Source: CAD feature listing. Evaluate the final solid. Frame: model axes, mm. A direction names the side the tool comes from. Coordinates: 2 decimals unless noted, no trailing zeros. Loops run counter-clockwise (first coordinate to the right, second up) from the corner with the lowest first, then second, coordinate; pieces in that order, holes last. Notation, with made-up numbers: (64, 65.5) -> (83, 65.5) arc R25 ccw to (83, 79.5) -> close; hole circle Ø3 at (-13, -1.75). An arc over 180 degrees is marked (long way). Answer as CSV lines item,"result".
from build123d import *

# Parameters (mm, degrees)
F0_R     = 0.825
F0_R_2   = 7.825
F0_W     = 2.625
F0_H     = 2.7
F1_DEPTH = 1.6
F0_R_3   = 6.175
F2_DEPTH = 13.8
F3_DEPTH = 11.65
F4_DEPTH = 3.1
F5_W     = 0.8
F5_H     = 0.8
F6_DEPTH = 2.4
F8_DEPTH = 0.8
F9_DEPTH = 5
F10_R    = 0.3


with BuildPart() as f1:
    # F0 (on Top) → F1 (new body)
    with BuildSketch(Plane.XY):
        Polygon((22.85, -10.65), (22.85, 10.65), (5.25, 10.65), (5.25, 7.95), (2.625, 7.95), (0, 7.95), (-2.625, 7.95), (-5.25, 7.95), (-5.25, 10.65), (-22.85, 10.65), (-22.85, -10.65), align=None)
        with Locations((-21.125, -8.675)):
            Circle(F0_R, mode=Mode.SUBTRACT)
        with BuildLine():
            ThreePointArc((-4.1107536526, -10.25), (-6.4607536526, -7.9), (-4.1107536526, -5.55))
            Line((-4.1107536526, -5.55), (4.1107536526, -5.55))
            ThreePointArc((4.1107536526, -5.55), (6.4607536526, -7.9), (4.1107536526, -10.25))
            Line((4.1107536526, -10.25), (-4.1107536526, -10.25))
        make_face(mode=Mode.SUBTRACT)
        with Locations((21.125, -8.675)):
            Circle(F0_R, mode=Mode.SUBTRACT)
        with Locations((-13.025, 0)):
            Circle(F0_R_2, mode=Mode.SUBTRACT)
        with Locations((-21.125, 8.675)):
            Circle(F0_R, mode=Mode.SUBTRACT)
        with Locations((13.025, 0)):
            Circle(F0_R_2, mode=Mode.SUBTRACT)
        with Locations((21.125, 8.675)):
            Circle(F0_R, mode=Mode.SUBTRACT)
        with Locations((-3.9375, 9.3)):
            Rectangle(F0_W, F0_H)
        with Locations((-1.3125, 9.3)):
            Rectangle(F0_W, F0_H)
        with Locations((1.3125, 9.3)):
            Rectangle(F0_W, F0_H)
        with Locations((3.9375, 9.3)):
            Rectangle(F0_W, F0_H)
    extrude(amount=F1_DEPTH)

    # F0 (on Top) → F2 (join)
    with BuildSketch(Plane.XY):
        with Locations((13.025, 0)):
            Circle(F0_R_2)
        with Locations((13.025, 0)):
            Circle(F0_R_3, mode=Mode.SUBTRACT)
        with Locations((-13.025, 0)):
            Circle(F0_R_2)
        with Locations((-13.025, 0)):
            Circle(F0_R_3, mode=Mode.SUBTRACT)
    extrude(amount=F2_DEPTH)

    # F0 (on Top) → F3 (join)
    with BuildSketch(Plane.XY):
        with Locations((-13.025, 0)):
            Circle(F0_R_3)
        with Locations((13.025, 0)):
            Circle(F0_R_3)
    extrude(amount=F3_DEPTH)

    # F0 (on Top) → F4 (join)
    with BuildSketch(Plane.XY):
        with Locations((-3.9375, 9.3)):
            Rectangle(F0_W, F0_H)
        with Locations((-1.3125, 9.3)):
            Rectangle(F0_W, F0_H)
        with Locations((1.3125, 9.3)):
            Rectangle(F0_W, F0_H)
        with Locations((3.9375, 9.3)):
            Rectangle(F0_W, F0_H)
    extrude(amount=-F4_DEPTH)

    # F5 (on face) → F6 (join)
    with BuildSketch(Plane(origin=(0, 0, -3.1), x_dir=(1, 0, 0), z_dir=(0, 0, -1))):
        with Locations((-3.9375, -9.3)):
            Rectangle(F5_W, F5_H)
        with Locations((-1.3125100119, -9.3)):
            Rectangle(F5_W, F5_H)
        with Locations((1.3124799761, -9.3)):
            Rectangle(F5_W, F5_H)
        with Locations((3.9374699642, -9.3)):
            Rectangle(F5_W, F5_H)
    extrude(amount=F6_DEPTH)

    # F7 (on face) → F8 (join)
    with BuildSketch(Plane(origin=(0, 0, -5.5), x_dir=(1, 0, 0), z_dir=(0, 0, -1))):
        Polygon((-4.3375, -8.9), (-4.3375, -9.7), (-4.3375, -16.8), (-3.5375, -16.8), (-3.5375, -9.7), (-3.5375, -8.9), align=None)
        Polygon((-1.7125100119, -8.9), (-1.7125100119, -9.7), (-1.7125100119, -16.8), (-0.9125100119, -16.8), (-0.9125100119, -9.7), (-0.9125100119, -8.9), align=None)
        Polygon((0.9124799761, -8.9), (0.9124799761, -9.7), (0.9124799761, -16.8), (1.7124799761, -16.8), (1.7124799761, -9.7), (1.7124799761, -8.9), align=None)
        Polygon((3.5374699642, -8.9), (3.5374699642, -9.7), (3.5374699642, -16.8), (4.3374699642, -16.8), (4.3374699642, -9.7), (4.3374699642, -8.9), align=None)
    extrude(amount=-F8_DEPTH)

    # F0 (on Top) → F9 (join)
    with BuildSketch(Plane.XY):
        with BuildLine():
            Line((4.1107536526, -5.55), (-4.1107536526, -5.55))
            ThreePointArc((-4.1107536526, -5.55), (-6.4607536526, -7.9), (-4.1107536526, -10.25))
            Line((-4.1107536526, -10.25), (4.1107536526, -10.25))
            ThreePointArc((4.1107536526, -10.25), (6.4607536526, -7.9), (4.1107536526, -5.55))
        make_face()
    extrude(amount=F9_DEPTH)

    # F10
    f10_edges = [f1.edges().sort_by_distance(p)[0] for p in [
        (-3.9375, 8.9, -5.5),
        (-1.31251, 8.9, -5.5),
        (1.31248, 8.9, -5.5),
        (3.93747, 8.9, -5.5),
        (3.93747, 9.7, -4.7),
        (1.31248, 9.7, -4.7),
        (-1.31251, 9.7, -4.7),
        (-3.9375, 9.7, -4.7),
    ]]
    fillet(f10_edges, radius=F10_R)


solid = f1.part
(1) Cut plane C-C (z = 10). Return the cut outline in (x, y) (3 decimals).
Computed values:
outline,"circle Ø15.65 at (-13.025, 0); circle Ø15.65 at (13.025, 0)"
(2) Cut plane A-A (z = 12.75). Return the cut outline in (x, y) (3 decimals).
Computed values:
outline,"circle Ø15.65 at (-13.025, 0); circle Ø15.65 at (13.025, 0); hole circle Ø12.35 at (-13.025, 0); hole circle Ø12.35 at (13.025, 0)"
(3) Pin query (flat end, axial travel): pin 1 Ø5 at (x, y) = (7.5, 10.5) entering from -Z; pin 2 Ø1.5 at (x, y) = (3.5, -4.5) entering from +Z; pin 3 Ø8 at (y, z) = (-4, 3.5) entering from -X; pin 4 Ø2 at (x, z) = (7, 1.5) entering from +Y. Return the tip coordinate at first contact, or that it passes through.
Computed values:
pin 1,"z = -3.1"
pin 2,"z = 1.6"
pin 3,"x = -22.85"
pin 4,"y = 10.65"
(4) Material intervals for L1, parallel to X at y = 2.5, z = 12.75; L2, parallel to Y at x = -4, z = -3.75; L3, parallel to Z at x = -16, y = -2.75, sorted ascending. Write a range as [from, to].
Computed values:
L1,"[-20.44, -18.67], [-7.38, -5.61], [5.61, 7.38], [18.67, 20.44]"
L2,"[8.9, 9.7]"
L3,"[0, 11.65]"
(5) Access query for faces 5 (the flat face through (1.712, 12, -5)), 6 (the flat face through (0, 9, -3.1)), 7 (the cylindrical face through (12.01, 7.76, 7.61)), 8 (the flat face through (0, -8, 5)). Directions: +Z, -Z, +X, -X, +Y, -Y. A direction counts if a zero-diameter tool reaches every point of the face in a straight line with its end or side. Return the directions, or none.
Computed values:
face 5,"-Z, +Y, -Y"
face 6,"none"
face 7,"+Z"
face 8,"+Z, -Y"
(6) Cut plane D-D (y = 0). Return the cut outline in (x, z), then the cut area to 3 significant figures.
Computed values:
outline,"(-22.85, 0) -> (22.85, 0) -> (22.85, 1.6) -> (20.85, 1.6) -> (20.85, 13.8) -> (19.2, 13.8) -> (19.2, 11.65) -> (6.85, 11.65) -> (6.85, 13.8) -> (5.2, 13.8) -> (5.2, 1.6) -> (-5.2, 1.6) -> (-5.2, 13.8) -> (-6.85, 13.8) -> (-6.85, 11.65) -> (-19.2, 11.65) -> (-19.2, 13.8) -> (-20.85, 13.8) -> (-20.85, 1.6) -> (-22.85, 1.6) -> close"
area,"402 mm^2"
(7) Cut plane B-B (y = 12.75). Return the cut outline in (x, z), then the cut area to 3 significant figures.
Computed values:
outline,"(-4.34, -5.5) -> (-3.54, -5.5) -> (-3.54, -4.7) -> (-4.34, -4.7) -> close; (-1.71, -5.5) -> (-0.91, -5.5) -> (-0.91, -4.7) -> (-1.71, -4.7) -> close; (0.91, -5.5) -> (1.71, -5.5) -> (1.71, -4.7) -> (0.91, -4.7) -> close; (3.54, -5.5) -> (4.34, -5.5) -> (4.34, -4.7) -> (3.54, -4.7) -> close"
area,"2.56 mm^2"
(8) Draft query along X for faces 1 (the flat face through (0, 7.95, -2)), 2 (the flat face through (5.25, 9, -2)), 3 (the cylindrical face through (-21.95, -8.64, 0.79)), 4 (the flat face through (-5.25, 9, -2)). Return one class per face: released by +X, released by -X, zero draft, split by the parting line, or undercut.
Computed values:
face 1,"zero draft"
face 2,"released by +X"
face 3,"undercut"
face 4,"released by -X"
